Design review of the part built by this model. Coordinates are the model's own, in mm. A direction names the side the tool comes from. Give positions to 0.01 mm unless a question says otherwise; leave off trailing zeros. Write each loop counter-clockwise with the first axis right and the second up, starting at its lowest first coordinate (ties: lowest second). Pieces come first, ordered by that corner, then holes.
```python
from build123d import *

# Parameters (mm, degrees)
ESQUISSE1_R                  = 6.35
ESQUISSE1_R_2                = 1.778
BOSS_EXTRU_1_DEPTH           = 6.35
BOSS_EXTRU_2_DEPTH           = 12.7
ENL_V_MAT_EXTRU_1_DEPTH      = 19.05
CONG_1_R                     = 6.35
ENL_V_MAT_EXTRU_2_REACH      = 45.845
ENL_V_MAT_EXTRU_2_END_RADIUS = 6.35
ESQUISSE5_R                  = 1.35255
ENL_V_MAT_EXTRU_3_DEPTH      = 44.844555452


with BuildPart() as part:
    # Esquisse1 → Boss.-Extru.1 (new body)
    with BuildSketch(Plane.XY):
        with BuildLine():
            Line((-10.2743, -7.465169758), (-10.2743, -32.258))
            Line((-10.2743, -32.258), (10.2743, -32.258))
            Line((10.2743, -32.258), (10.2743, -7.465169758))
            ThreePointArc((10.2743, -7.465169758), (0, 12.7), (-10.2743, -7.465169758))
        make_face()
        Circle(ESQUISSE1_R, mode=Mode.SUBTRACT)
        with Locations((0, 9.779)):
            Circle(ESQUISSE1_R_2, mode=Mode.SUBTRACT)
        with Locations((6.914797213, 6.914797213)):
            Circle(ESQUISSE1_R_2, mode=Mode.SUBTRACT)
        with Locations((9.779, 0)):
            Circle(ESQUISSE1_R_2, mode=Mode.SUBTRACT)
        with Locations((6.914797213, -6.914797213)):
            Circle(ESQUISSE1_R_2, mode=Mode.SUBTRACT)
        with Locations((0, -9.779)):
            Circle(ESQUISSE1_R_2, mode=Mode.SUBTRACT)
        with Locations((-6.914797213, -6.914797213)):
            Circle(ESQUISSE1_R_2, mode=Mode.SUBTRACT)
        with Locations((-9.779, 0)):
            Circle(ESQUISSE1_R_2, mode=Mode.SUBTRACT)
        with Locations((-6.914797213, 6.914797213)):
            Circle(ESQUISSE1_R_2, mode=Mode.SUBTRACT)
    extrude(amount=BOSS_EXTRU_1_DEPTH)

    # Esquisse2 → Boss.-Extru.2 (add)
    with BuildSketch(Plane.XZ.offset(32.258)):
        with BuildLine():
            Line((-10.2743, 10.1092), (-10.2743, 6.35))
            Line((-10.2743, 6.35), (10.2743, 6.35))
            Line((10.2743, 6.35), (10.2743, 10.1092))
            ThreePointArc((10.2743, 10.1092), (8.9042183, 15.235225455), (5.159375, 18.994136134))
            Line((5.159375, 18.994136134), (5.159375, 23.7236))
            Line((5.159375, 23.7236), (-5.159375, 23.7236))
            Line((-5.159375, 23.7236), (-5.159375, 18.994136134))
            ThreePointArc((-5.159375, 18.994136134), (-8.9042183, 15.235225455), (-10.2743, 10.1092))
        make_face()
    extrude(amount=-BOSS_EXTRU_2_DEPTH)

    # Esquisse3 → Enlèv. mat.-Extru.1 (cut)
    with BuildSketch(Plane.XZ.offset(32.258)):
        with BuildLine():
            Line((-0.396875, 18.036771916), (-0.396875, 23.7236))
            Line((-0.396875, 23.7236), (0.396875, 23.7236))
            Line((0.396875, 23.7236), (0.396875, 18.036771916))
            ThreePointArc((0.396875, 18.036771916), (0, 2.1717), (-0.396875, 18.036771916))
        make_face()
    extrude(amount=-ENL_V_MAT_EXTRU_1_DEPTH, mode=Mode.SUBTRACT)

    # Congé1
    cong_1_edges = [part.edges().sort_by_distance(p)[0] for p in [
        (-5.159375, -25.908, 18.994136134),
        (5.159375, -25.908, 18.994136134),
    ]]
    fillet(cong_1_edges, radius=CONG_1_R)

    # Enlèv. mat.-Extru.2: up to this cylinder (the profile starts outside it)
    enl_v_mat_extru_2_end = Plane(origin=(11.509375, -25.908, 22.105100867), z_dir=(0, -1, 0)) * Cylinder(ENL_V_MAT_EXTRU_2_END_RADIUS, 105.39, mode=Mode.PRIVATE)
    # Esquisse4 → Enlèv. mat.-Extru.2 (cut, up to the surface)
    with BuildSketch(Plane(origin=(5.159375, 0, 0), x_dir=(0, 0, -1), z_dir=(1, 0, 0)), mode=Mode.PRIVATE) as enl_v_mat_extru_2_sk1:
        with BuildLine():
            Line((-19.1516, -21.1455), (-19.1516, -30.6705))
            ThreePointArc((-19.1516, -30.6705), (-21.4376, -32.9565), (-23.7236, -30.6705))
            Line((-23.7236, -30.6705), (-23.7236, -21.1455))
            ThreePointArc((-23.7236, -21.1455), (-21.4376, -18.8595), (-19.1516, -21.1455))
        make_face()
    enl_v_mat_extru_2_tool1 = extrude(enl_v_mat_extru_2_sk1.sketch, amount=ENL_V_MAT_EXTRU_2_REACH, mode=Mode.PRIVATE) - enl_v_mat_extru_2_end
    add(enl_v_mat_extru_2_tool1.solids().sort_by_distance((5.159375, -25.908, 21.4376))[0], mode=Mode.SUBTRACT)
    add(enl_v_mat_extru_2_tool1.solids().sort_by_distance((5.159375, -25.908, 21.4376))[1], mode=Mode.SUBTRACT)

    # Esquisse5 → Enlèv. mat.-Extru.3 (cut, through all)
    with BuildSketch(Plane(origin=(5.159375, 0, 0), x_dir=(0, 0, -1), z_dir=(1, 0, 0))):
        with Locations(Location((-21.415375, -22.733, 0), (0, 0, 120.660154312))):
            Circle(ESQUISSE5_R)
        with Locations(Location((-21.415375, -29.083, 0), (0, 0, 239.339845688))):
            Circle(ESQUISSE5_R)
    extrude(amount=-ENL_V_MAT_EXTRU_3_DEPTH, mode=Mode.SUBTRACT)


solid = part.part
```
(1) Tool access review of faces 1 (the face through (-5.159, -26, 23)), 2 (the face through (10.274, -20, 4)), 3 (the face through (0, -7, 6.35)): name each direction out of +Z, -Z, +X, -X, +Y, -Y from which nothing blocks a thin tool from reaching the whole face with its end or side.
Resolved:
face 1: +Z, -X, +Y, -Y
face 2: +Z, -Z, +X, -Y
face 3: +Z, +X, -X, +Y
(2) Consider section C-C, the plane z = 8.5. Give the boundary of the cut face in (x, y).
Resolved:
outline: (-10.27, -32.26) - (-7.77, -32.26) - (-7.77, -19.56) - (-10.27, -19.56) - close; (7.77, -32.26) - (10.27, -32.26) - (10.27, -19.56) - (7.77, -19.56) - close
(3) Mouldability with a two-part tool opening along Z and no side actions: class faces 4 (the face through (-9.43, -26, 14.19)), 5 (the face through (5.159, -26, 21)), 6 (the face through (2.811, -28.157, 22.402)) as pulls with the +Z half, pulls with the -Z half, needs draft (parallel to the pull), parting line crosses it, or undercut.
Resolved:
face 4: pulls with the +Z half
face 5: needs draft
face 6: undercut
(4) Clearance check with flat-ended pins moving along their axes: P1, Ø1.4, axis at y = -26.5, z = 21, coming from the +X side; P2, Ø4.5, axis at x = 0, y = 9.779, coming from the +Z side; P3, Ø8, axis at x = 4, z = 14, coming from the -Y side; P4, Ø8, axis at y = -17.5, z = 5, coming from the -X side. State where each tip first meets the part, or that it passes through.
Resolved:
P1: stops at x = 5.16
P2: stops at z = 6.35
P3: stops at y = -32.26
P4: stops at x = -10.27
(5) Consider section A-A, the plane y = 0. Give the boundary of the cut face in (x, z), then the cut area to 3 significant figures.
Resolved:
outline: (-12.7, 0) - (-11.56, 0) - (-11.56, 6.35) - (-12.7, 6.35) - close; (-8, 0) - (-6.35, 0) - (-6.35, 6.35) - (-8, 6.35) - close; (6.35, 0) - (8, 0) - (8, 6.35) - (6.35, 6.35) - close; (11.56, 0) - (12.7, 0) - (12.7, 6.35) - (11.56, 6.35) - close
area: 35.5 mm2
(6) Consider section D-D, the plane x = 9.5. Give the boundary of the cut face in (y, z).
Resolved:
outline: (-32.26, 0) - (-1.76, 0) - (-1.76, 6.35) - (-19.56, 6.35) - (-19.56, 14.02) - (-32.26, 14.02) - close; (1.76, 0) - (8.43, 0) - (8.43, 6.35) - (1.76, 6.35) - close
(7) Consider section B-B, the plane x = 2.5. Give the boundary of the cut face in (y, z).
Resolved:
outline: (-32.26, 0) - (-5.84, 0) - (-5.84, 6.35) - (-13.21, 6.35) - (-13.21, 2.58) - (-32.26, 2.58) - close; (-32.26, 17.64) - (-19.56, 17.64) - (-19.56, 23.72) - (-32.26, 23.72) - close; (5.84, 0) - (12.45, 0) - (12.45, 6.35) - (5.84, 6.35) - close; hole circle Ø2.71 at (-29.08, 21.42); hole circle Ø2.71 at (-22.73, 21.42)
(8) To check wall thickness, follow L1, parallel to Y at x = 0, z = 2.75; L2, parallel to Y at x = -1, z = 5.25; L3, parallel to Y at x = 5, z = 20.25. State the ranges of each line that lie inside material, in increasing order.
Resolved:
L1: y = -13.21 to -11.56, -8 to -6.35, 6.35 to 8, 11.56 to 12.7
L2: y = -13.21 to -11.25, -8.31 to -6.27, 6.27 to 8.31, 11.25 to 12.66
L3: y = -32.26 to -29.77, -28.4 to -23.42, -22.05 to -19.56
